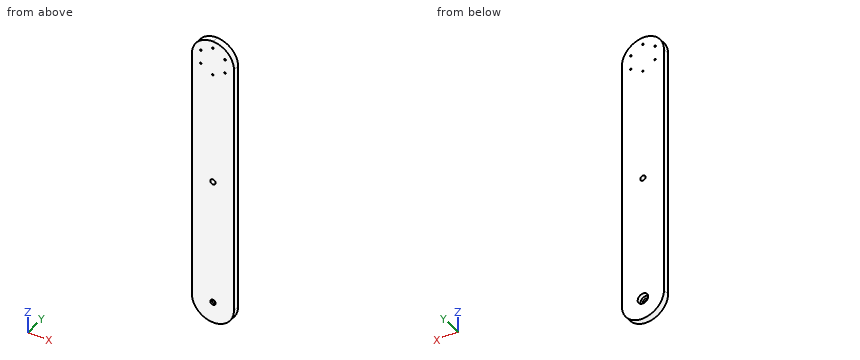
Autodesk Inventor part; units mm, degrees
ref_plane "YZ Plane" through (0, 0, 0) normal (1, 0, 0) x (0, 1, 0)
ref_plane "XZ Plane" through (0, 0, 0) normal (0, 1, 0) x (-1, 0, 0)
ref_plane "XY Plane" through (0, 0, 0) normal (0, 0, 1) x (1, 0, 0)
sketch "Szkic1" plane through (0, 0, 0) normal (0, 1, 0) x (-1, 0, 0)
  line L0 (-20, 140) -> (20, 140)
  line L1 (20, 140) -> (20, -120)
  line L2 (0, -140) -> (0, -140)
  line L3 (-20, -120) -> (-20, 140)
  arc A0 (0, -140) -> (20, -120) centre (0, -120) ccw
  arc A1 (-20, -120) -> (0, -140) centre (0, -120) ccw
  circle A2 centre (0, -120) radius 5
  circle A3 centre (0, 0) radius 2.5
  point P0 (20, -120)
  point P1 (0, -140)
  point P2 (-20, -120)
  point P3 (20, -120)
  point P4 (-20, -120)
  point P5 (0, -140)
  dimension "d3" = 20
  dimension "d4" = 20
  dimension "d9" = 5
extrude "Wyciągnięcie proste2" add sketch "Szkic1" along normal blind 6
sketch "Szkic2" plane through (0, 6, 0) normal (0, 1, 0) x (1, 0, 0)
  line L0 (0, -106.7) -> (11.5181, -113.35)
  line L1 (11.5181, -113.35) -> (11.5181, -126.65)
  line L2 (11.5181, -126.65) -> (0, -133.3)
  line L3 (0, -133.3) -> (-11.5181, -126.65)
  line L4 (-11.5181, -126.65) -> (-11.5181, -113.35)
  line L5 (-11.5181, -113.35) -> (0, -106.7)
  circle A0 centre (-11.5181, -113.35) radius 0.75
  circle A1 centre (0, -106.7) radius 0.75
  circle A2 centre (11.5181, -113.35) radius 0.75
  circle A3 centre (11.5181, -126.65) radius 0.75
  circle A4 centre (0, -133.3) radius 0.75
  circle A5 centre (-11.5181, -126.65) radius 0.75
  point P0 (0, 0)
  point P1 (-20.5841, -116.7396)
  point P2 (0, -120)
  point P3 (0, -120)
  point P4 (0, -120)
  dimension "d12" = 1.5
  dimension "d13" = 1.5
  dimension "d14" = 1.5
  dimension "d15" = 1.5
  dimension "d16" = 1.5
  dimension "d17" = 1.5
extrude "Wyciągnięcie proste3" cut sketch "Szkic2" against normal blind 6 contours L5 A1 L0 | L0 A1 L5 | A2 L1 L0 | L0 L1 A2 | A0 L4 L5 | L5 L4 A0 | A3 L2 L1 | L1 L2 A3 | A5 L3 L4 | L4 L3 A5 | A4 L3 L2 | L2 L3 A4
sketch "Szkic3" plane through (0, 0, 0) normal (0, -1, 0) x (1, 0, 0)
  circle A0 centre (0, -120) radius 5
  circle A1 centre (0, -120) radius 2.5
  point P0 (0, 0)
  dimension "d30" = 10
  dimension "d31" = 5
extrude "Wyciągnięcie proste4" add sketch "Szkic3" against normal blind 2
fillet "Zaokrąglenie1" radius 20 1 edges at (20, 3, 140)
fillet "Zaokrąglenie2" radius 20 1 edges at (-20, 3, 140)
properties part number "GroundArm"
Geometry: final body of the model. Coordinates: model frame, mm. Coordinates: 2 decimals unless noted, no trailing zeros. Loops run counter-clockwise (first coordinate to the right, second up) from the corner with the lowest first, then second, coordinate; pieces in that order, holes last. Notation, with made-up numbers: (18, 10.5) -> (51, 10.5) arc R15 cw to (51, 37.5) -> close; hole circle Ø9 at (-5.5, 7). An arc over 180 degrees is marked (long way). Use a Markdown table: item, result. Add a question column.
(1) Section query A-A, the plane y = 3.45. State how many separate pieces and enclosed holes the cut face has, plus the area to 3 significant figures.
(2) Line query: line 1 along Z through (x, y) = (0, 3.1); line 2 along X through (y, z) = (4.6, 113.35); line 3 along Z through (x, y) = (-4, 5.55). Output: solid intervals per line, ascending.
(3) Pin query (flat end, axial travel): pin 1 Ø1.5 at (x, y) = (9, 3) entering from -Z; pin 2 Ø2 at (x, y) = (14, 4) entering from -Z. Return the tip coordinate at first contact, or that it passes through.
(4) Section query B-B, the plane z = 0. Return loops of the section in (x, y).
Answer:
| question | item | result |
|---|---|---|
| 1 | separate pieces | 1 |
| 1 | enclosed holes | 8 |
| 1 | area | 10,700 mm^2 |
| 2 | line 1 | z = -140 to -125, -115 to -2.5, 2.5 to 105.95, 107.45 to 132.55, 134.05 to 140 |
| 2 | line 2 | x = -20 to -12.27, -10.77 to 10.77, 12.27 to 20 |
| 2 | line 3 | z = -139.6 to -123, -117 to 139.6 |
| 3 | pin 1 | stops at z = -138.22 |
| 3 | pin 2 | stops at z = -135.2 |
| 4 | outline | (-20, 0) -> (-2.5, 0) -> (-2.5, 6) -> (-20, 6) -> close; (2.5, 0) -> (20, 0) -> (20, 6) -> (2.5, 6) -> close |
